Here's how the part is built. I have some questions about the finished solid (model axes, mm). Round coordinates to 2 decimals unless told otherwise and drop trailing zeros. Order: outer loops, then holes, each group sorted by start corner. A loop starts at its lowest first (then second) coordinate and runs counter-clockwise, first axis right, second up. Notation, with made-up numbers: (63, -18.75) - (82, -18.75) arc R27 cw to (82, 18.25) - close; hole circle Ø6 at (52, 82.5). An arc over 180 degrees is marked (long way). Answer as a JSON object with one key per item and string values.
```python
from build123d import *

# Parameters (mm, degrees)
BOSS_EXTRUDE1_DEPTH      = 50
BOSS_EXTRUDE1_DEPTH_BACK = 50
BOSS_EXTRUDE2_START      = 50
BOSS_EXTRUDE2_DEPTH      = 5
BOSS_EXTRUDE3_START      = -55
BOSS_EXTRUDE3_DEPTH      = 5


with BuildPart() as part:
    # Sketch2 → Boss-Extrude1 (new, two sides: drawn at the far end of the back side and taken through both)
    with BuildSketch(Plane(origin=(0, 0, 0), x_dir=(0, 0, -1), z_dir=(1, 0, 0)).offset(-BOSS_EXTRUDE1_DEPTH_BACK)):
        Polygon((-147.070290747, 193.522440667), (-147.070290747, 218.522440667), (-177.070290747, 231.022440667), (-217.070290747, 231.022440667), (-217.070290747, 181.022440667), (-177.070290747, 181.022440667), align=None)
    extrude(amount=BOSS_EXTRUDE1_DEPTH + BOSS_EXTRUDE1_DEPTH_BACK)

    # Sketch3 → Boss-Extrude2 (add)
    with BuildSketch(Plane(origin=(0, 0, 0), x_dir=(0, 0, -1), z_dir=(1, 0, 0)).offset(BOSS_EXTRUDE2_START)):
        with BuildLine():
            Line((-207.070290747, 203.022440667), (-187.070290747, 203.022440667))
            ThreePointArc((-187.070290747, 203.022440667), (-184.070290747, 206.022440667), (-187.070290747, 209.022440667))
            Line((-187.070290747, 209.022440667), (-207.070290747, 209.022440667))
            ThreePointArc((-207.070290747, 209.022440667), (-210.070290747, 206.022440667), (-207.070290747, 203.022440667))
        make_face()
    extrude(amount=BOSS_EXTRUDE2_DEPTH)

    # Sketch3<2> → Boss-Extrude3 (add)
    with BuildSketch(Plane(origin=(0, 0, 0), x_dir=(0, 0, -1), z_dir=(1, 0, 0)).offset(BOSS_EXTRUDE3_START)):
        with BuildLine():
            Line((-207.070290747, 203.022440667), (-187.070290747, 203.022440667))
            ThreePointArc((-187.070290747, 203.022440667), (-184.070290747, 206.022440667), (-187.070290747, 209.022440667))
            Line((-187.070290747, 209.022440667), (-207.070290747, 209.022440667))
            ThreePointArc((-207.070290747, 209.022440667), (-210.070290747, 206.022440667), (-207.070290747, 203.022440667))
        make_face()
    extrude(amount=BOSS_EXTRUDE3_DEPTH)


solid = part.part
```
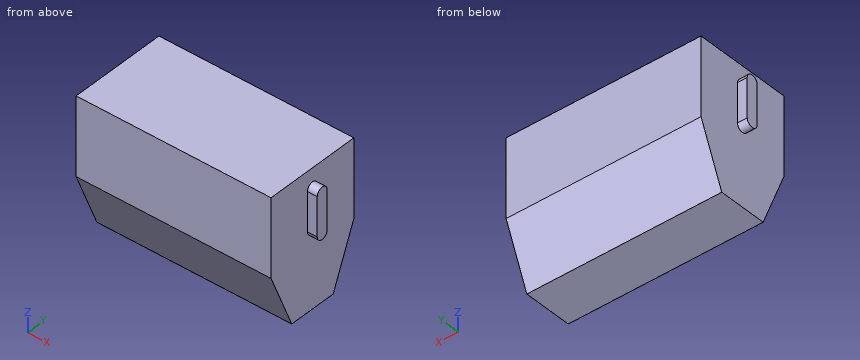
1. If I drill on L1, parallel to X at y = 217.5, z = 161.5; L2, parallel to Y at x = -14, z = 165; L3, parallel to Z at x = 4.5, y = 228.5, over which ranges is the centre line in solid material (lowest first)? Write a range as [from, to].
Responses:
{"L1": "[-50, 50]", "L2": "[186.05, 225.99]", "L3": "[171.02, 217.07]"}
2. Imagine slicing it at B-B (x = 12.5). List the corners of the cut face in (y, z) for me, plus the area to 4 significant figures.
Responses:
{"outline": "(181.02, 177.07) - (193.52, 147.07) - (218.52, 147.07) - (231.02, 177.07) - (231.02, 217.07) - (181.02, 217.07) - close", "area": "3,125 mm2"}
3. Imagine slicing it at D-D (z = 178.5). List the corners of the cut face in (x, y) for me.
Responses:
{"outline": "(-50, 181.02) - (50, 181.02) - (50, 231.02) - (-50, 231.02) - close"}
4. Imagine slicing it at A-A (z = 201). List the corners of the cut face in (x, y) for me, plus the area to 3 significant figures.
Responses:
{"outline": "(-55, 203.02) - (-50, 203.02) - (-50, 181.02) - (50, 181.02) - (50, 203.02) - (55, 203.02) - (55, 209.02) - (50, 209.02) - (50, 231.02) - (-50, 231.02) - (-50, 209.02) - (-55, 209.02) - close", "area": "5,060 mm2"}
5. Imagine slicing it at C-C (y = 207). List the corners of the cut face in (x, z) for me.
Responses:
{"outline": "(-55, 184.23) - (-50, 184.23) - (-50, 147.07) - (50, 147.07) - (50, 184.23) - (55, 184.23) - (55, 209.91) - (50, 209.91) - (50, 217.07) - (-50, 217.07) - (-50, 209.91) - (-55, 209.91) - close"}
6. For P1, Ø10, axis at y = 215.5, z = 180, coming from the -X side; P2, Ø1.5, axis at x = -51.5, z = 196, coming from the +Y side; P3, Ø5.5, axis at x = -53.5, z = 200, coming from the -Y side; P4, Ø25, axis at y = 200.5, z = 181.5, coming from the -X side, each with a flat end and sliding along its axis, tell me the tip position at first contact or that it passes through.
Responses:
{"P1": "x = -50", "P2": "y = 209.02", "P3": "y = 203.02", "P4": "x = -55"}
